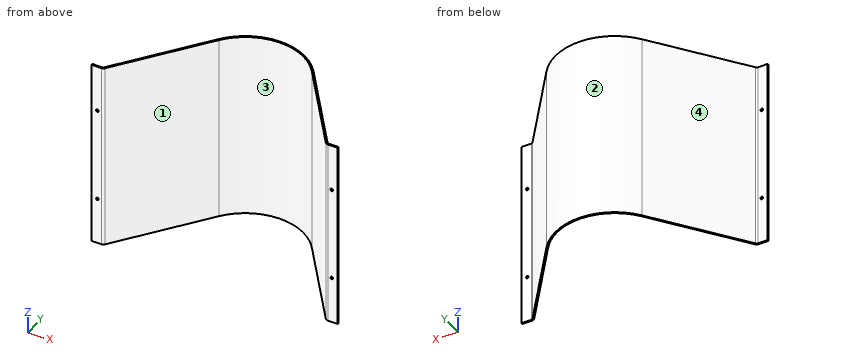
from build123d import *

# Parameters (mm, degrees)
F1_DEPTH = 609.6
F2_T     = 2.38125
F3_W     = 393.7
F3_H     = 155.575
F4_DEPTH = 179.0405708
F5_R     = 2.15265
F6_DEPTH = 2.38125


# Not quite as in the source:
# - a shell that OpenCascade refuses in one call is made with other operations: the cavity is built on its own and cut out


with BuildPart() as f1:
    # F0 (on Top) → F1 (new body)
    with BuildSketch(Plane.XY):
        with BuildLine():
            Line((15.875, 0), (0, 0))
            Line((0, 0), (0, -2.38125))
            Line((0, -2.38125), (393.7, -2.38125))
            Line((393.7, -2.38125), (393.7, 0))
            Line((393.7, 0), (377.825, 0))
            ThreePointArc((377.825, 0), (376.4007720387, 0.337360186), (375.2792072647, 1.2777482116))
            Line((375.2792072647, 1.2777482116), (273.096492423, 138.389761864))
            ThreePointArc((273.096492423, 138.389761864), (196.85, 176.6583208), (120.603507577, 138.389761864))
            Line((120.603507577, 138.389761864), (18.4207927353, 1.2777482116))
            ThreePointArc((18.4207927353, 1.2777482116), (17.2992279613, 0.337360186), (15.875, 0))
        make_face()
    extrude(amount=F1_DEPTH)

    # F2: shell of thickness 2.38125, made by hand


with BuildPart() as f2_core1:
    # F2_t2: copy of F1
    add(f1.part)

    # the walls: a layer under each face that stays
    f2_faces = [f2_core1.faces().sort_by_distance(p)[0] for p in [
        (196.85, 176.6583208, 304.8),
        (69.5121501562, 69.8337550378, 304.8),
        (17.2992279613, 0.337360186, 304.8),
        (7.9375, 0, 304.8),
        (0, -1.190625, 304.8),
        (393.7, -1.190625, 304.8),
        (385.7625, 0, 304.8),
        (376.4007720387, 0.337360186, 304.8),
        (324.1878498438, 69.8337550378, 304.8),
        (196.85, 87.1385354, 0),
        (196.85, 87.1385354, 609.6),
    ]]
    thicken(f2_faces, amount=-F2_T, mode=Mode.SUBTRACT)


with BuildPart() as f1_1:
    add(f1.part)

    # what is left inside the walls is the cavity
    f2_cavity = [f2_core1.part.solids().sort_by_distance(p)[0] for p in [
        (196.85, -2.357438, 405.60625),
    ]]
    add(f2_cavity, mode=Mode.SUBTRACT)

    # F3 (on face) → F4 (cut, through all)
    with BuildSketch(Plane.XZ.offset(2.38125)):
        with Locations((196.85, 531.8125)):
            Rectangle(F3_W, F3_H)
        with Locations((196.85, 77.7875)):
            Rectangle(F3_W, F3_H)
    extrude(amount=-F4_DEPTH, mode=Mode.SUBTRACT)

    # F5 (on face) → F6 (cut, through all)
    with BuildSketch(Plane.XZ.offset(2.38125)):
        with Locations((384.175, 230.1875)):
            Circle(F5_R)
        with Locations((384.175, 379.4125)):
            Circle(F5_R)
        with Locations((9.525, 379.4125)):
            Circle(F5_R)
        with Locations((9.525, 230.1875)):
            Circle(F5_R)
    extrude(amount=-F6_DEPTH, mode=Mode.SUBTRACT)


solid = f1_1.part
The model under review builds one solid part; all positions refer to its coordinate system, in mm. Face numbers are marked on the shaded views. Give positions to 0.01 mm unless a question says otherwise; leave off trailing zeros. Order: outer loops, then holes, each group sorted by start corner. A loop starts at its lowest first (then second) coordinate and runs counter-clockwise, first axis right, second up. Notation, with made-up numbers: M -24,3 L 17,3 A20 ccw 17,39 Z; hole C 62.25,3 d3. An arc over 180 degrees is marked long. Use one line per item in the form item = value. Start each with the question number.
Item 1: The part is to be moulded in two halves that separate along X. For the marked faces 1, 2, 3 and 4, say which applies: pulls with the +X half, pulls with the -X half, needs draft (parallel to the pull), parting line crosses it, or undercut.
Item 2: We need section C-C on x = 45. Give the boundary of the cut face in (y, z) (3 decimals).
Item 3: We need section A-A on y = 10. Give the boundary of the cut face in (x, z) (3 decimals), plus the area to 3 significant figures.
Item 4: To check wall thickness, follow line 1 along X through (y, z) = (25.5, 292); line 2 along X through (y, z) = (63.5, 411); line 3 along Y through (x, z) = (203, 261). State the ranges of each line that lie inside material, in increasing order. Write a range as from..to.
Item 5: Insertion check: pin 1 Ø17.5 at (x, z) = (8.5, 249) entering from +Y; pin 2 Ø5.5 at (x, z) = (384.18, 379.41) entering from +Y; pin 3 Ø1 at (x, z) = (98, 337) entering from +Y. Each pin has a flat end and moves straight along its axis. Give the tip position at first contact, or say it passes through.
Completed:
q1.face_1 = undercut
q1.face_2 = parting line crosses it
q1.face_3 = undercut
q1.face_4 = pulls with the -X half
q2.outline = M 32.958,155.575 L 36.943,155.575 L 36.943,454.025 L 32.958,454.025 Z
q3.outline = M 24.921,155.575 L 27.891,155.575 L 27.891,454.025 L 24.921,454.025 Z; M 365.809,155.575 L 368.779,155.575 L 368.779,454.025 L 365.809,454.025 Z
q3.area = 1,770 mm²
q4.line_1 = 36.47..39.44, 354.26..357.23
q4.line_2 = 64.79..67.76, 325.94..328.91
q4.line_3 = 174.07..176.46
q5.pin_1 = 0.31
q5.pin_2 = 0
q5.pin_3 = 108.73
